Source: CAD feature listing. Evaluate the final solid. Frame: model axes, mm. Face numbers are marked on the shaded views. Round coordinates to 2 decimals unless told otherwise and drop trailing zeros. Write each loop counter-clockwise with the first axis right and the second up, starting at its lowest first coordinate (ties: lowest second). Pieces come first, ordered by that corner, then holes. Notation, with made-up numbers: M 20.5,52 L 60.5,52 A26 ccw 60.5,69 Z; hole C 16.5,-39 d9. An arc over 180 degrees is marked long. Answer in a Markdown table with one row per item.
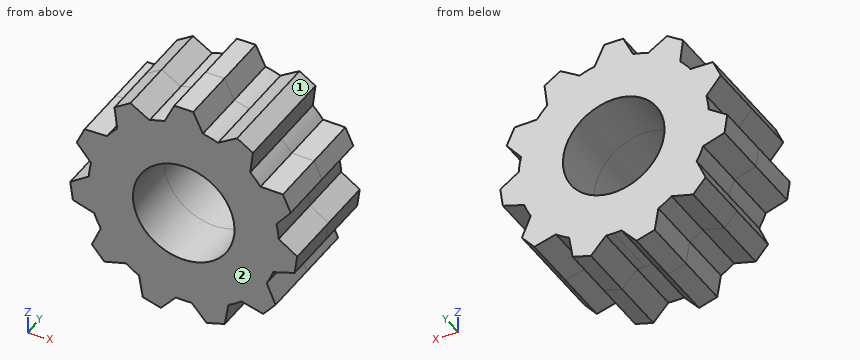
from build123d import *
from build123d.topology import SkipClean

# Parameters (mm, degrees)
SKETCH1_R            = 4.5
BOSS_EXTRUDE1_DEPTH  = 4.999999999999969
SKETCH12_R           = 8.425
SKETCH12_R_2         = 4.5
BOSS_EXTRUDE6_DEPTH  = 5
BOSS_EXTRUDE9_DEPTH  = 5
CIRPATTERN2_COUNT    = 11
BOSS_EXTRUDE10_START = 5
SKETCH17_R           = 8.425
SKETCH17_R_2         = 4.5
BOSS_EXTRUDE10_DEPTH = 5
BOSS_EXTRUDE11_DEPTH = 5
SKETCH19_R           = 4.5
CUT_EXTRUDE1_DEPTH   = 10


with BuildPart() as part:
    # Sketch1 → Boss-Extrude1 (new body)
    with BuildSketch(Plane(origin=(0, 0, 0), x_dir=(1, 0, 0), z_dir=(0, 1, 0))):
        with Locations(Location((0, 0, 0), (0, 0, 270))):
            Circle(SKETCH1_R)
    extrude(amount=BOSS_EXTRUDE1_DEPTH)

    # Sketch19 → Cut-Extrude1 (cut)
    with BuildSketch(Plane.XZ):
        with Locations(Location((0, 0, 0), (0, 0, 270))):
            Circle(SKETCH19_R)
    extrude(amount=-CUT_EXTRUDE1_DEPTH, mode=Mode.SUBTRACT)


with BuildPart() as body_2:
    # Sketch12 → Boss-Extrude6 (new body)
    with BuildSketch(Plane(origin=(0, 5, 0), x_dir=(-1, 0, 0), z_dir=(0, -1, 0))):
        with Locations(Location((0, 0, 0), (0, 0, 90))):
            Circle(SKETCH12_R)
        with Locations(Location((0, 0, 0), (0, 0, 270))):
            Circle(SKETCH12_R_2, mode=Mode.SUBTRACT)
    extrude(amount=BOSS_EXTRUDE6_DEPTH)



with BuildPart() as body_3:
    # Sketch13 → Boss-Extrude9 (new body)
    with BuildSketch(Plane.XZ):
        with BuildLine():
            Line((1.700000000000002, 8.251704369401512), (0.84, 10.039921563438629))
            Line((0.84, 10.039921563438629), (-0.84, 10.039921563438629))
            Line((-0.84, 10.039921563438629), (-1.6999999999999977, 8.251704369401512))
            ThreePointArc((-1.6999999999999977, 8.251704369401514), (2.39e-15, 8.425), (1.7000000000000024, 8.251704369401512))
        make_face()
    extrude(amount=-BOSS_EXTRUDE9_DEPTH)


with BuildPart() as cirpattern2_1:
    # CirPattern2: pattern copy
    add(body_3.part.rotate(Axis((-9e-17, 0, -3.9e-16), (0, 1, 0)), 1 * 360 / CIRPATTERN2_COUNT))


with BuildPart() as cirpattern2_2:
    # CirPattern2: pattern copy
    add(body_3.part.rotate(Axis((-9e-17, 0, -3.9e-16), (0, 1, 0)), 2 * 360 / CIRPATTERN2_COUNT))


with BuildPart() as cirpattern2_3:
    # CirPattern2: pattern copy
    add(body_3.part.rotate(Axis((-9e-17, 0, -3.9e-16), (0, 1, 0)), 3 * 360 / CIRPATTERN2_COUNT))


with BuildPart() as cirpattern2_4:
    # CirPattern2: pattern copy
    add(body_3.part.rotate(Axis((-9e-17, 0, -3.9e-16), (0, 1, 0)), 4 * 360 / CIRPATTERN2_COUNT))


with BuildPart() as cirpattern2_5:
    # CirPattern2: pattern copy
    add(body_3.part.rotate(Axis((-9e-17, 0, -3.9e-16), (0, 1, 0)), 5 * 360 / CIRPATTERN2_COUNT))


with BuildPart() as cirpattern2_6:
    # CirPattern2: pattern copy
    add(body_3.part.rotate(Axis((-9e-17, 0, -3.9e-16), (0, 1, 0)), 6 * 360 / CIRPATTERN2_COUNT))


with BuildPart() as cirpattern2_7:
    # CirPattern2: pattern copy
    add(body_3.part.rotate(Axis((-9e-17, 0, -3.9e-16), (0, 1, 0)), 7 * 360 / CIRPATTERN2_COUNT))


with BuildPart() as cirpattern2_8:
    # CirPattern2: pattern copy
    add(body_3.part.rotate(Axis((-9e-17, 0, -3.9e-16), (0, 1, 0)), 8 * 360 / CIRPATTERN2_COUNT))


with BuildPart() as cirpattern2_9:
    # CirPattern2: pattern copy
    add(body_3.part.rotate(Axis((-9e-17, 0, -3.9e-16), (0, 1, 0)), 9 * 360 / CIRPATTERN2_COUNT))


with BuildPart() as cirpattern2_10:
    # CirPattern2: pattern copy
    add(body_3.part.rotate(Axis((-9e-17, 0, -3.9e-16), (0, 1, 0)), 10 * 360 / CIRPATTERN2_COUNT))


with BuildPart() as body_2_1:
    with SkipClean():  # the faces are left unmerged after this step: merging them gives an invalid solid
        add(body_2.part)

        add(body_3.part)  # Boss-Extrude10 merges body 3

        add(cirpattern2_2.part)  # Boss-Extrude10 merges CirPattern2_2

        add(cirpattern2_3.part)  # Boss-Extrude10 merges CirPattern2_3

        add(cirpattern2_4.part)  # Boss-Extrude10 merges CirPattern2_4

        add(cirpattern2_5.part)  # Boss-Extrude10 merges CirPattern2_5

        add(cirpattern2_6.part)  # Boss-Extrude10 merges CirPattern2_6

        add(cirpattern2_7.part)  # Boss-Extrude10 merges CirPattern2_7

        add(cirpattern2_8.part)  # Boss-Extrude10 merges CirPattern2_8

        add(cirpattern2_9.part)  # Boss-Extrude10 merges CirPattern2_9

        add(cirpattern2_10.part)  # Boss-Extrude10 merges CirPattern2_10
        # Sketch17 → Boss-Extrude10 (add)
        # profile 1 of 11: a face of its own
        with BuildSketch(Plane.XZ.offset(BOSS_EXTRUDE10_START)):
            Circle(SKETCH17_R)
            with Locations(Location((0, 0, 0), (0, 0, 90))):
                Circle(SKETCH17_R_2, mode=Mode.SUBTRACT)
        # profile 2 of 11: a face of its own
        with BuildSketch(Plane.XZ.offset(BOSS_EXTRUDE10_START)):
            with BuildLine():
                ThreePointArc((-1.6999999999999988, 8.251704369401518), (2.05e-15, 8.425000000000002), (1.7000000000000028, 8.251704369401514))
                Line((1.7000000000000024, 8.251704369401512), (0.8400000000000013, 10.039921563438629))
                Line((0.8400000000000013, 10.039921563438629), (-0.8400000000000009, 10.039921563438629))
                Line((-0.8400000000000009, 10.039921563438629), (-1.6999999999999984, 8.251704369401514))
            make_face()
        # profile 3 of 11: a face of its own
        with BuildSketch(Plane.XZ.offset(BOSS_EXTRUDE10_START)):
            with BuildLine():
                ThreePointArc((-5.891339201488175, 6.022686062962995), (-4.554898887063417, 7.087561014102698), (-3.0310771898621596, 7.860864842312031))
                Line((-3.03107718986216, 7.860864842312031), (-4.72133843366936, 8.9002577712534))
                Line((-4.72133843366936, 8.9002577712534), (-6.134644368825746, 7.991981197927994))
                Line((-6.134644368825746, 7.991981197927994), (-5.891339201488176, 6.022686062962995))
            make_face()
        # profile 4 of 11: a face of its own
        with BuildSketch(Plane.XZ.offset(BOSS_EXTRUDE10_START)):
            with BuildLine():
                Line((-9.481582495875129, 3.4066432707159575), (-8.212219832717508, 1.8815074857999516))
                ThreePointArc((-8.21221983271751, 1.8815074857999512), (-7.663649560861826, 3.4998714845408747), (-6.7998087885111005, 4.974256270005318))
                Line((-6.7998087885111, 4.974256270005317), (-8.783685274031965, 4.934825022911553))
                Line((-8.783685274031965, 4.934825022911553), (-9.481582495875129, 3.4066432707159575))
            make_face()
        # profile 5 of 11: a face of its own
        with BuildSketch(Plane.XZ.offset(BOSS_EXTRUDE10_START)):
            with BuildLine():
                Line((-9.818185174144725, -2.260279824757259), (-7.925778691831604, -2.8570364240079513))
                ThreePointArc((-7.925778691831604, -2.857036424007951), (-8.339245647846854, -1.1990025124524568), (-8.409649141960784, 0.5083564783872193))
                Line((-8.409649141960784, 0.5083564783872193), (-10.057274102443852, -0.5973798023972904))
                Line((-10.057274102443852, -0.5973798023972905), (-9.818185174144725, -2.260279824757259))
            make_face()
        # profile 6 of 11: a face of its own
        with BuildSketch(Plane.XZ.offset(BOSS_EXTRUDE10_START)):
            with BuildLine():
                Line((-7.037583431604806, -7.20958004624413), (-5.1229588171653475, -6.688491456048056))
                ThreePointArc((-5.1229588171653475, -6.688491456048055), (-6.367190163934598, -5.517201683489059), (-7.349485312579329, -4.118942903243587))
                Line((-7.34948531257933, -4.118942903243588), (-8.137749464632893, -5.93992076132898))
                Line((-8.137749464632893, -5.93992076132898), (-7.037583431604806, -7.20958004624413))
            make_face()
        # profile 7 of 11: a face of its own
        with BuildSketch(Plane.XZ.offset(BOSS_EXTRUDE10_START)):
            with BuildLine():
                Line((-2.022598674718725, -9.869889543506861), (-0.6936357151463852, -8.396397709415234))
                ThreePointArc((-0.6936357151463853, -8.396397709415236), (-2.3735967913889944, -8.08372830270216), (-3.955911825435684, -7.4385070161543965))
                Line((-3.9559118254356838, -7.438507016154395), (-3.634546870391086, -9.39657884801327))
                Line((-3.634546870391086, -9.39657884801327), (-2.022598674718725, -9.869889543506861))
            make_face()
        # profile 8 of 11: a face of its own
        with BuildSketch(Plane.XZ.offset(BOSS_EXTRUDE10_START)):
            with BuildLine():
                Line((3.6345468703912207, -9.396578848013215), (3.955911825435787, -7.438507016154339))
                ThreePointArc((3.955911825435787, -7.438507016154339), (2.3735967913891054, -8.083728302702124), (0.6936357151465026, -8.396397709415222))
                Line((0.6936357151465024, -8.396397709415224), (2.022598674718867, -9.86988954350683))
                Line((2.022598674718867, -9.86988954350683), (3.6345468703912207, -9.396578848013215))
            make_face()
        # profile 9 of 11: a face of its own
        with BuildSketch(Plane.XZ.offset(BOSS_EXTRUDE10_START)):
            with BuildLine():
                Line((5.122958817165441, -6.688491456047983), (7.037583431604909, -7.209580046244029))
                Line((7.037583431604909, -7.209580046244029), (8.137749464632977, -5.939920761328863))
                Line((8.137749464632977, -5.939920761328863), (7.349485312579388, -4.118942903243486))
                ThreePointArc((7.349485312579388, -4.118942903243488), (6.367190163934675, -5.51720168348897), (5.122958817165442, -6.6884914560479825))
            make_face()
        # profile 10 of 11: a face of its own
        with BuildSketch(Plane.XZ.offset(BOSS_EXTRUDE10_START)):
            with BuildLine():
                ThreePointArc((8.425, 5e-16), (8.299256306401244, -1.4501619773870813), (7.925778691831642, -2.8570364240078403))
                Line((7.925778691831642, -2.8570364240078403), (9.818185174144755, -2.260279824757118))
                Line((9.818185174144755, -2.260279824757118), (10.05727410244386, -0.5973798023971462))
                Line((10.05727410244386, -0.597379802397146), (8.409649141960777, 0.5083564783873361))
                ThreePointArc((8.409649141960777, 0.508356478387336), (8.42116141102341, 0.25429410038423766), (8.425, 5e-16))
            make_face()
        # profile 11 of 11: a face of its own
        with BuildSketch(Plane.XZ.offset(BOSS_EXTRUDE10_START)):
            with BuildLine():
                ThreePointArc((6.79980878851103, 4.974256270005415), (7.663649560861776, 3.499871484540982), (8.21221983271748, 1.8815074858000667))
                Line((8.21221983271748, 1.8815074858000667), (9.481582495875081, 3.4066432707160943))
                Line((9.481582495875081, 3.4066432707160943), (8.783685274031892, 4.934825022911679))
                Line((8.783685274031892, 4.934825022911679), (6.799808788511031, 4.974256270005414))
            make_face()
        extrude(amount=-BOSS_EXTRUDE10_DEPTH)


    add(cirpattern2_1.part)  # Boss-Extrude11 merges CirPattern2_1
    # Sketch18 → Boss-Extrude11 (add)
    with BuildSketch(Plane.XZ):
        with BuildLine():
            Line((6.1346443688256285, 7.991981197928084), (4.721338433669231, 8.900257771253472))
            Line((4.721338433669231, 8.900257771253472), (3.031077189862048, 7.860864842312075))
            ThreePointArc((3.031077189862048, 7.860864842312075), (4.554898887063315, 7.087561014102763), (5.891339201488088, 6.022686062963079))
            Line((5.891339201488088, 6.022686062963079), (6.1346443688256285, 7.991981197928084))
        make_face()
    extrude(amount=BOSS_EXTRUDE11_DEPTH)


solid = body_2_1.part
Q1. Section D-D (z = 5.5). Return loops of the section in (x, y), and give its area (3 significant figures).
Solutions:
| item | result |
|---|---|
| outline | M -6.38,-5 L 6.38,-5 L 6.38,5 L -6.38,5 Z |
| area | 128 mm2 |
Q2. Section A-A (z = -1.25). Return loops of the section in (x, y).
Solutions:
| item | result |
|---|---|
| outline | M -9.96,-5 L -4.32,-5 L -4.32,5 L -9.96,5 Z; M 4.32,-5 L 9.96,-5 L 9.96,5 L 4.32,5 Z |
Q3. Pull-direction query (X, two-part tool) for the marked faces 1 and 2; classes: pulls with the +X half, pulls with the -X half, needs draft (parallel to the pull), parting line crosses it, or undercut.
Solutions:
| item | result |
|---|---|
| face 1 | pulls with the +X half |
| face 2 | needs draft |
Q4. Material intervals for probe 1 along X at (y, z) = (-0.25, 3.25); probe 2 along X at (y, z) = (1.5, 4); probe 3 along Z at (x, y) = (-8, 3), sorted ascending.
Solutions:
| item | result |
|---|---|
| probe 1 | x = -9.35 to -3.11, 3.11 to 9.35 |
| probe 2 | x = -9.21 to -2.06, 2.06 to 9.21 |
| probe 3 | z = -6.1 to -5.62, -2.83 to 4.95 |
Q5. Section B-B (z = -3.5). Return loops of the section in (x, y).
Solutions:
| item | result |
|---|---|
| outline | M -7.66,-5 L -2.83,-5 L -2.83,5 L -7.66,5 Z; M 2.83,-5 L 7.66,-5 L 7.66,5 L 2.83,5 Z |
Q6. Section C-C (z = -5.5). Return loops of the section in (x, y), and give its area (3 significant figures).
Solutions:
| item | result |
|---|---|
| outline | M -7.95,-5 L 7.95,-5 L 7.95,5 L -7.95,5 Z |
| area | 159 mm2 |
Q7. Contact query for flat-ended pins moving along their axis: pin 1 Ø6 at (x, y) = (5, 3) entering from +Z; pin 2 Ø1.5 at (y, z) = (1, 1.5) entering from +X; pin 3 Ø5.5 at (x, z) = (0, 0) entering from -Y; pin 4 Ø11.5 at (x, z) = (0, 0) entering from +Y. Output: stop coordinate, or through.
Solutions:
| item | result |
|---|---|
| pin 1 | stops at z = 8.9 |
| pin 2 | stops at x = 8.52 |
| pin 3 | passes through |
| pin 4 | stops at y = 5 |
